Here's the drawing with two shaded views (mm, measured from the low corner). I have some questions. A direction names the side the tool comes from. Round coordinates to 2 decimals unless told otherwise and drop trailing zeros. Use one line per item in the form item = value. Start each with the question number.
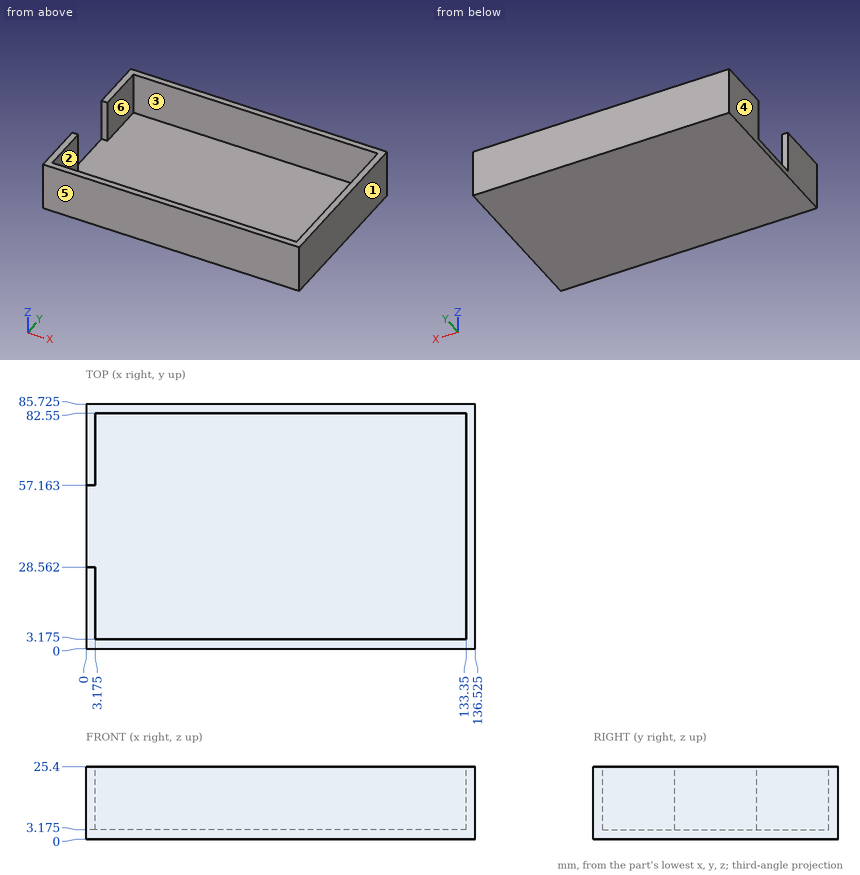
1. Will these pins go through, and if not, where does the flat tip stop? pin 1 (6.5 mm diameter, centred on y = 44, z = 14.5, fed in from -X); pin 2 (1 mm diameter, centred on x = 59, y = 20, fed in from +Z) (3 decimals).
2. If we mould it in two halves opening along X, with no side actions, what happens to the marked faces 3, 4, 5 and 6? For each: pulls with the +X half, pulls with the -X half, needs draft (parallel to the pull), parting line crosses it, or undercut.
3. Which directions (+Z, -Z, +X, -X, +Y, -Y) give clear straight access to the entire face, cutting with the end or side of a thin tool? Please do the marked faces 1 and 2.
4. Please list where this line runs through material, in increasing order: line 1 along Z through (x, y) = (75, 55.5) (1 decimal).
Model answer:
q1.pin_1 = 133.35
q1.pin_2 = 3.175
q2.face_3 = undercut
q2.face_4 = pulls with the -X half
q2.face_5 = needs draft
q2.face_6 = undercut
q3.face_1 = +Z, -Z, +X, +Y, -Y
q3.face_2 = +Z
q4.line_1 = 0 to 3.2
